Can you work these out from the model? Positions are in its coordinate system, mm. A direction names the side the tool comes from. Give positions to 0.01 mm unless a question says otherwise; leave off trailing zeros. Order: outer loops, then holes, each group sorted by start corner. A loop starts at its lowest first (then second) coordinate and runs counter-clockwise, first axis right, second up. Notation, with made-up numbers: (24.5, 60.5) -> (44.5, 60.5) arc R14 cw to (44.5, 84.5) -> close; hole circle Ø1 at (-1.75, 76). An arc over 180 degrees is marked (long way). Answer as CSV lines item,"result".
Autodesk Inventor part; units mm, degrees
ref_plane "YZ Plane" through (0, 0, 0) normal (1, 0, 0) x (0, 1, 0)
ref_plane "XZ Plane" through (0, 0, 0) normal (0, 1, 0) x (-1, 0, 0)
ref_plane "XY Plane" through (0, 0, 0) normal (0, 0, 1) x (1, 0, 0)
sketch "Esquisse1" plane through (0, 0, 0) normal (1, 0, 0) x (0, 1, 0)
  line L0 (3, 0) -> (23, 0)
  line L1 (23, 0) -> (23, -12)
  line L2 (23, -12) -> (26, -12)
  line L3 (26, -12) -> (26, -23)
  line L4 (29, -35) -> (23, -35)
  line L5 (23, -35) -> (23, -18)
  line L6 (23, -18) -> (6, -18)
  line L7 (6, -18) -> (6, -35)
  line L8 (6, -35) -> (0, -35)
  line L9 (26, -23) -> (29, -23)
  line L10 (29, -23) -> (29, -35)
  line L11 (3, 0) -> (3, -13)
  line L12 (3, -13) -> (0, -13)
  line L13 (0, -13) -> (0, -35)
  point P0 (0, 0)
  dimension "d0" = 35
  dimension "d2" = 17
  dimension "d4" = 17
  dimension "d6" = 3
  dimension "d7" = 12
  dimension "d8" = 12
  dimension "d10" = 3
  dimension "d34" = 13
  dimension "d35" = 3
  dimension "d36" = 29
  dimension "d37" = 6
  dimension "d38" = 0
  dimension "d44" = 0
extrude "Extrusion1" add sketch "Esquisse1" along normal blind 20
sketch "Esquisse2" plane through (0, 29, -23) normal (0, 1, 0) x (1, 0, 0)
  line L0 (0, 12) -> (20, 12)
  line L1 (20, 12) -> (20, 0)
  point P0 (0, -23)
  point P1 (9, 6)
  dimension "d20" = 6
  dimension "d21" = 11
hole "Perçage1" at (9, 29, -29) direction (0, -1, 0) diameter 4 end through all
sketch "Esquisse3" plane through (0, 23, 0) normal (0, 1, 0) x (1, 0, 0)
  line L0 (0, 0) -> (20, 0)
  line L1 (0, 12) -> (0, 0)
  point P0 (3, 6)
  dimension "d29" = 6
  dimension "d30" = 3
hole "Perçage2" at (3, 23, -6) direction (0, -1, 0) diameter 3.5 end through all
pattern_linear "Réseau rectangulaire1" count 2 spacing 14 along (1, 0, 0) of "Perçage2"
chamfer "Chanfrein1" distance 5 angle 45 2 edges at (0, 14.5, -18) (20, 14.5, -18)
fillet "Congé1" radius 5 6 edges at (0, 26, -35) (20, 26, -35) (0, 3, -35) (20, 3, -35) (20, 13, 0) (0, 13, 0)
fillet "Congé2" radius 5 1 edges at (10, 26, -23)
properties part number "support_avant_3DPrint"
Item 1: Please list where these lines run through material, in increasing order: line 1 along Y through (x, z) = (12.25, -30.5); line 2 along Z through (x, y) = (9, 5); line 3 along X through (y, z) = (3, -29).
Numbers:
line 1,"y = 0 to 6, 23 to 29"
line 2,"z = -35 to -31, -27 to 0"
line 3,"x = 0 to 7, 11 to 20"
Item 2: Imagine slicing it at D-D, the plane z = -6. Please give me the cut outline in (x, y), then the cut area to 3 significant figures.
Numbers:
outline,"(0, 3) -> (1.25, 3) -> (1.25, 23) -> (0, 23) -> close; (4.75, 3) -> (15.25, 3) -> (15.25, 23) -> (4.75, 23) -> close; (18.75, 3) -> (20, 3) -> (20, 23) -> (18.75, 23) -> close"
area,"260 mm²"
Item 3: For faces 1 (the flat face through (10, 2, -13)), 2 (the flat face through (17, 15, -16)), 3 (the flat face through (10, 23, -6)), 4 (the flat face through (0, 11, -12)), 5 (the cylindrical face through (1, 3, -33)), which set-ups out of +Z, -Z, +X, -X, +Y, -Y let a thin tool reach every point of the face, with its end or its side?
Numbers:
face 1,"+Z, +X, -X, -Y"
face 2,"-Z, +X"
face 3,"+Z, +X, -X, +Y"
face 4,"+Z, -Z, -X, +Y, -Y"
face 5,"-Z, -X, +Y, -Y"
Item 4: We'd pull the mould along Y, two halves only. Please class faces 6 (the flat face through (10, 0, -24)), 7 (the flat face through (10, 26, -35)), 8 (the flat face through (3, 15, -16)), 9 (the flat face through (10, 26, -15)): released by +Y, released by -Y, zero draft, split by the parting line, or undercut.
Numbers:
face 6,"released by -Y"
face 7,"zero draft"
face 8,"undercut"
face 9,"released by +Y"
Item 5: Imagine slicing it at C-C, the plane y = 5.5. Please give me the cut outline in (x, z).
Numbers:
outline,"(0, -30) arc R5 ccw to (5, -35) -> (15, -35) arc R5 ccw to (20, -30) -> (20, -5) arc R5 ccw to (15, 0) -> (5, 0) arc R5 ccw to (0, -5) -> close; hole circle Ø3.5 at (3, -6); hole circle Ø4 at (9, -29); hole circle Ø3.5 at (17, -6)"
Item 6: Imagine slicing it at A-A, the plane x = 9. Please give me the cut outline in (y, z).
Numbers:
outline,"(0, -35) -> (6, -35) -> (6, -31) -> (0, -31) -> close; (0, -27) -> (6, -27) -> (6, -18) -> (23, -18) -> (23, -27) -> (29, -27) -> (29, -23) arc R5 cw to (26, -18.42) -> (26, -12) -> (23, -12) -> (23, 0) -> (3, 0) -> (3, -13) -> (0, -13) -> close; (23, -35) -> (29, -35) -> (29, -31) -> (23, -31) -> close"
Item 7: For pin 1 (4 mm diameter, centred on x = 7, y = 17.5, fed in from -Z); pin 2 (1.9 mm diameter, centred on x = 10.5, z = -15, fed in from +Y); pin 3 (3.5 mm diameter, centred on x = 9.5, z = -4, fed in from +Y), each with a flat end and sliding along its axis, tell me the tip position at first contact or that it passes through.
Numbers:
pin 1,"stops at z = -18"
pin 2,"stops at y = 26"
pin 3,"stops at y = 23"
Item 8: Imagine slicing it at B-B, the plane z = -26. Please give me the cut outline in (x, y), then the cut area to 3 significant figures.
Numbers:
outline,"(0, 0) -> (20, 0) -> (20, 6) -> (0, 6) -> close; (0, 23) -> (20, 23) -> (20, 29) -> (0, 29) -> close"
area,"240 mm²"
